Check sheet for the modelled part. Datum: model origin and axes. Units: mm. Face numbers are marked on the shaded views. A direction names the side the tool comes from. Give positions to 0.01 mm unless a question says otherwise; leave off trailing zeros. Write each loop counter-clockwise with the first axis right and the second up, starting at its lowest first coordinate (ties: lowest second). Pieces come first, ordered by that corner, then holes. Notation, with made-up numbers: (81, 30.25) -> (121, 30.25) arc R27 ccw to (121, 56.25) -> close; hole circle Ø4 at (77.5, -36.5). An arc over 180 degrees is marked (long way). Answer as a JSON object with one key per item and string values.
Solid Edge part; units mm, degrees
sketch "Sketch1" plane through (0, 0, 0) normal (1, 0, 0) x (0, 1, 0)
  line L0 (-26, 37.5) -> (-26, 0)
  line L1 (-26, -37.5) -> (-26, 0)
  line L2 (-16, -37.5) -> (-26, -37.5)
  line L3 (0, -37.5) -> (-16, -37.5)
  line L4 (0, -37.5) -> (16, -37.5)
  line L5 (16, -37.5) -> (26, -37.5)
  line L6 (26, -37.5) -> (26, 0)
  line L7 (26, 37.5) -> (26, 0)
  line L8 (16, 37.5) -> (26, 37.5)
  line L9 (0, 37.5) -> (16, 37.5)
  line L10 (0, 37.5) -> (-16, 37.5)
  line L11 (-16, 37.5) -> (-26, 37.5)
extrude "Protrusion1" add sketch "Sketch1" along normal blind 15
sketch "Sketch2" plane through (0, 0, 0) normal (1, 0, 0) x (0, 1, 0)
  circle A0 centre (-16, 27.5006) radius 5
  circle A1 centre (-16, -27.5006) radius 5
  circle A2 centre (16, -27.5006) radius 5
  circle A3 centre (16, 27.5006) radius 5
extrude "ExtrudedCutout_1" cut sketch "Sketch2" along normal blind 26.9909
sketch "Sketch3" plane through (0, 0, 0) normal (1, 0, 0) x (0, 1, 0)
  line L0 (6, -32.5) -> (6, -12.5)
  line L1 (6, -12.5) -> (-6, -12.5)
  line L2 (-6, -12.5) -> (-6, -32.5)
  line L3 (0, -32.5) -> (-6, -32.5)
  line L4 (0, -32.5) -> (6, -32.5)
extrude "ExtrudedProtrusion_2" add sketch "Sketch3" against normal blind 10
sketch "Sketch4" plane through (-5, -6, -22.5) normal (0, -1, 0) x (-1, 0, 0)
  line L0 (15, -20) -> (35, -20)
  line L1 (5, -10) -> (5, 10)
  arc A0 (5, 10) -> (35, -20) centre (5, -20) cw
  arc A1 (5, -10) -> (15, -20) centre (5, -20) cw
extrude "ExtrudedProtrusion_4" add sketch "Sketch4" against normal blind 12
sketch "Sketch5" plane through (-30, 0, -2.5) normal (0, 0, 1) x (0, 1, 0)
  line L0 (6, -10) -> (6, 10)
  line L1 (6, 10) -> (-6, 10)
  line L2 (-6, 10) -> (-6, -10)
  line L3 (-6, -10) -> (6, -10)
extrude "ExtrudedProtrusion_5" add sketch "Sketch5" along normal blind 10
sketch "Sketch6" plane through (0, 0, 0) normal (0, -1, 0) x (1, 0, 0)
  line L0 (-20, 30.5) -> (-40, 30.5)
  line L1 (-40, 30.5) -> (-40, 38.5)
  line L2 (-40, 38.5) -> (-20, 38.5)
  line L3 (-20, 38.5) -> (-20, 30.5)
revolve "RevolvedCutout1" cut sketch "Sketch6" angle 360 about axis through (-15.4193, 0, 22.5) along (-1, 0, 0)
sketch "Sketch7" plane through (0, 0, 0) normal (0, -1, 0) x (1, 0, 0)
  line L0 (-40, 30.5) -> (-40, 38.5)
  line L1 (-40, 38.5) -> (-20, 38.5)
  line L2 (-20, 38.5) -> (-20, 30.5)
  line L3 (-20, 30.5) -> (-40, 30.5)
revolve "RevolvedProtrusion1" add sketch "Sketch7" angle 360 about axis through (-15.4193, 0, 22.5) along (-1, 0, 0)
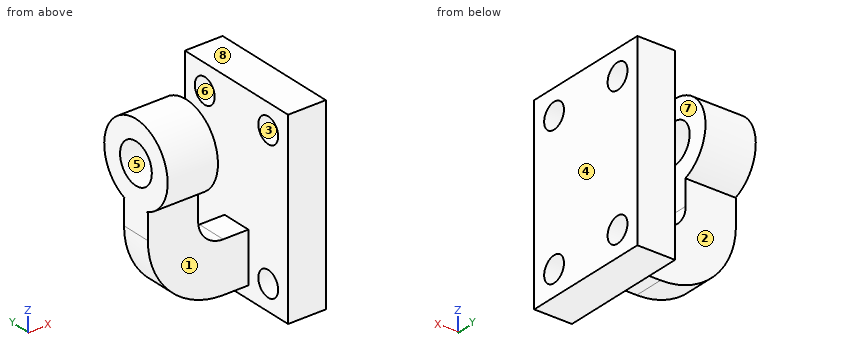
1. Sectioned sample at A-A, the plane y = 0. Enter the section's corners in (x, z), plus the area to 3 significant figures.
Determined:
{"outline": "(-40, -2.5) arc R30 ccw to (-10, -32.5) -> (0, -32.5) -> (0, -37.5) -> (15, -37.5) -> (15, 37.5) -> (0, 37.5) -> (0, -12.5) -> (-10, -12.5) arc R10 cw to (-20, -2.5) -> (-20, 14.5) -> (-40, 14.5) -> close; (-40, 30.5) -> (-20, 30.5) -> (-20, 38.5) -> (-40, 38.5) -> close", "area": "2,450 mm^2"}
2. Access from +Z, -Z, +X, -X, +Y, -Y to the whole of each face (thin tool, end or side, straight path). Record for the marked faces 5, 6, 7 and 8.
Determined:
{"face 5": "-X", "face 6": "+X", "face 7": "+Z, +Y, -Y", "face 8": "+Z, +X, +Y, -Y"}
3. Mould release check, pull along Y, two halves, no side actions. Record for the marked faces 1, 2, 3 and 4: released by +Y, released by -Y, zero draft, split by the parting line, or undercut.
Determined:
{"face 1": "released by -Y", "face 2": "released by +Y", "face 3": "undercut", "face 4": "zero draft"}
4. Go/stop test with flat-tipped pins: P1, Ø3, axis at y = -0.5, z = 27.5, coming from the -X side; P2, Ø4.5, axis at x = 10, y = -2.5, coming from the +Z side; P3, Ø3, axis at x = -6, y = 0.5, coming from the -Z side. Record where each tip stops, or that it passes through.
Determined:
{"P1": "x = 0", "P2": "z = 37.5", "P3": "z = -32.5"}
5. Scan lines: L1, parallel to Z at x = 4.25, y = 16; L2, parallel to X at y = 6, z = 29.5; L3, parallel to Y at x = -15.5, z = -13. Record each from-to range of solid material in increasing order. Write a range as [from, to].
Determined:
{"L1": "[-37.5, -32.5], [-22.5, 22.5], [32.5, 37.5]", "L2": "[-40, -20], [0, 15]", "L3": "[-6, 6]"}
6. Sectioned sample at B-B, the plane z = -10. Enter the section's corners in (x, y), plus the area to 3 significant figures.
Determined:
{"outline": "(-39.05, -6) -> (-16.61, -6) -> (-16.61, 6) -> (-39.05, 6) -> close; (0, -26) -> (15, -26) -> (15, 26) -> (0, 26) -> close", "area": "1,050 mm^2"}
7. Sectioned sample at C-C, the plane x = -22. Enter the section's corners in (y, z).
Determined:
{"outline": "(-6, -30) -> (6, -30) -> (6, 7.5) -> (5.57, 7.5) arc R16 ccw (long way) to (-5.57, 7.5) -> (-6, 7.5) -> close; hole circle Ø16 at (0, 22.5)"}
8. Sectioned sample at D-D, the plane y = 17.5. Enter the section's corners in (x, z).
Determined:
{"outline": "(0, -37.5) -> (15, -37.5) -> (15, -32.27) -> (0, -32.27) -> close; (0, -22.73) -> (15, -22.73) -> (15, 22.73) -> (0, 22.73) -> close; (0, 32.27) -> (15, 32.27) -> (15, 37.5) -> (0, 37.5) -> close"}
